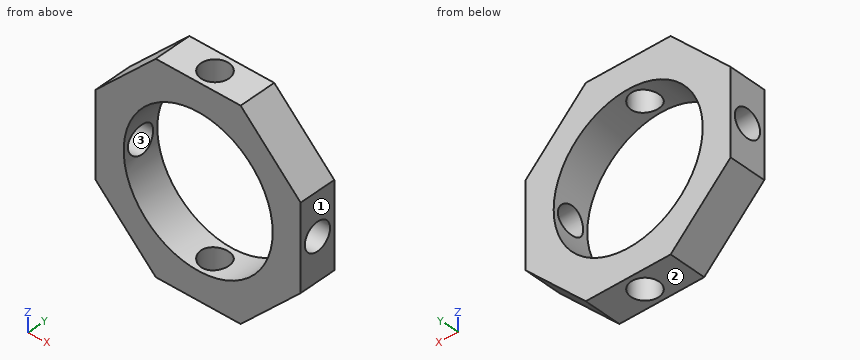
```python
from build123d import *

# Parameters (mm, degrees)
SKETCH2_R           = 50.8
BOSS_EXTRUDE1_DEPTH = 25.4
SKETCH3_R           = 9.525
CUT_EXTRUDE1_DEPTH  = 140.7
SKETCH4_R           = 9.525
CUT_EXTRUDE2_DEPTH  = 140.7


with BuildPart() as part:
    # Sketch2 → Boss-Extrude1 (new body)
    with BuildSketch(Plane(origin=(0, 0, 0), x_dir=(1, 0, 0), z_dir=(0, 1, 0))):
        Polygon((69.85, 28.932817332), (28.932817332, 69.85), (-28.932817332, 69.85), (-69.85, 28.932817332), (-69.85, -28.932817332), (-28.932817332, -69.85), (28.932817332, -69.85), (69.85, -28.932817332), align=None)
        Circle(SKETCH2_R, mode=Mode.SUBTRACT)
    extrude(amount=BOSS_EXTRUDE1_DEPTH)

    # Sketch3 → Cut-Extrude1 (cut, through all)
    with BuildSketch(Plane.XY.offset(69.85)):
        with Locations((0, 12.7)):
            Circle(SKETCH3_R)
    extrude(amount=-CUT_EXTRUDE1_DEPTH, mode=Mode.SUBTRACT)

    # Sketch4 → Cut-Extrude2 (cut, through all)
    with BuildSketch(Plane.ZY.offset(69.85)):
        with Locations((0, 12.7)):
            Circle(SKETCH4_R)
    extrude(amount=-CUT_EXTRUDE2_DEPTH, mode=Mode.SUBTRACT)


solid = part.part
```
Model file for the job. Use its own axes, mm. Face numbers are marked on the shaded views. Give positions to 0.01 mm unless a question says otherwise; leave off trailing zeros. Order: outer loops, then holes, each group sorted by start corner. A loop starts at its lowest first (then second) coordinate and runs counter-clockwise, first axis right, second up.
1) Saw through at A-A, the plane x = -20.5. Write the cut outline in (y, z).
2) Wall check: probe 1 along Y at (x, z) = (64.5, 0) (3 decimals); probe 2 along Y at (x, z) = (3, 57.5); probe 3 along Z at (x, y) = (16, 20.25). Give the ranges that are in metal, low to high.
3) Saw through at D-D, the plane z = 0. Write the cut outline in (x, y) (3 decimals).
4) Mould opens along Z. For the marked faces 1, 2 and 3 say: +Z half, -Z half, draft (parallel to the pull), parting line (faces both ways), or undercut.
5) Saw through at B-B, the plane x = 0. Write the cut outline in (y, z) (3 decimals).
6) Pin check, flat tips, straight feed: pin 1 (11.5 mm diameter, centred on x = 0, y = 12.7, fed in from +Z); pin 2 (4 mm diameter, centred on y = 11, z = 7.5, fed in from -X); pin 3 (6 mm diameter, centred on x = 45.5, y = 22.5, fed in from -Z); pin 4 (1.5 mm diameter, centred on y = 16, z = -31, fed in from -X). Stop position of each tip, or through.
7) Saw through at C-C, the plane y = 12.7. Write the cut outline in (x, z) (3 decimals), then the cut area to 3 significant figures.
Computed:
1. outline: (0, -69.85) - (25.4, -69.85) - (25.4, -46.48) - (0, -46.48) - close; (0, 46.48) - (25.4, 46.48) - (25.4, 69.85) - (0, 69.85) - close
2. probe 1: y = 0 to 3.175, 22.225 to 25.4
2. probe 2: y = 0 to 3.66, 21.74 to 25.4
2. probe 3: z = -69.85 to -48.21, 48.21 to 69.85
3. outline: (-69.85, 0) - (-50.8, 0) - (-50.8, 3.175) - (-69.85, 3.175) - close; (-69.85, 22.225) - (-50.8, 22.225) - (-50.8, 25.4) - (-69.85, 25.4) - close; (50.8, 0) - (69.85, 0) - (69.85, 3.175) - (50.8, 3.175) - close; (50.8, 22.225) - (69.85, 22.225) - (69.85, 25.4) - (50.8, 25.4) - close
4. face 1: draft
4. face 2: -Z half
4. face 3: undercut
5. outline: (0, -69.85) - (3.175, -69.85) - (3.175, -50.8) - (0, -50.8) - close; (0, 50.8) - (3.175, 50.8) - (3.175, 69.85) - (0, 69.85) - close; (22.225, -69.85) - (25.4, -69.85) - (25.4, -50.8) - (22.225, -50.8) - close; (22.225, 50.8) - (25.4, 50.8) - (25.4, 69.85) - (22.225, 69.85) - close
6. pin 1: passes through
6. pin 2: stops at x = -69.85
6. pin 3: stops at z = -56.28
6. pin 4: stops at x = -68.53
7. outline: (-69.85, -28.933) - (-28.933, -69.85) - (-9.525, -69.85) - (-9.525, -49.899) arc R50.8 cw to (-49.899, -9.525) - (-69.85, -9.525) - close; (-69.85, 9.525) - (-49.899, 9.525) arc R50.8 cw to (-9.525, 49.899) - (-9.525, 69.85) - (-28.933, 69.85) - (-69.85, 28.933) - close; (9.525, -69.85) - (28.933, -69.85) - (69.85, -28.933) - (69.85, -9.525) - (49.899, -9.525) arc R50.8 cw to (9.525, -49.899) - close; (9.525, 49.899) arc R50.8 cw to (49.899, 9.525) - (69.85, 9.525) - (69.85, 28.933) - (28.933, 69.85) - (9.525, 69.85) - close
7. area: 6,590 mm2
